from build123d import *

# Parameters (mm, degrees)
F0_R     = 2.05
F0_W     = 5.2
F0_H     = 2.15
F1_DEPTH = 2.9
F0_H_2   = 2.9
F2_DEPTH = 8


with BuildPart() as f1:
    # F0 (on Front) → F1 (new body)
    with BuildSketch(Plane.XZ):
        with BuildLine():
            Line((25.45, 4.556051), (4.65, 4.556051))
            ThreePointArc((4.65, 4.556051), (0, 6.51), (-4.65, 4.556051))
            Line((-4.65, 4.556051), (-16.95, 4.556051))
            ThreePointArc((-16.95, 4.556051), (-35.532978, 0), (-16.95, -4.556051))
            Line((-16.95, -4.556051), (-4.65, -4.556051))
            ThreePointArc((-4.65, -4.556051), (0, -6.51), (4.65, -4.556051))
            Line((4.65, -4.556051), (25.45, -4.556051))
            ThreePointArc((25.45, -4.556051), (31.693638, -7.699915), (37.907447, -4.497499))
            Line((37.907447, -4.497499), (37.907447, 0))
            Line((37.907447, 0), (37.907447, 4.497499))
            ThreePointArc((37.907447, 4.497499), (31.693638, 7.699915), (25.45, 4.556051))
        make_face()
        Polygon((-32.329781, 0), (-25.682978, 6.646804), (-19.036174, 0), (-25.682978, -6.646804), align=None, mode=Mode.SUBTRACT)
        with Locations((31.657447, 0)):
            Circle(F0_R, mode=Mode.SUBTRACT)
        Polygon((45.207447, 4.497499), (37.907447, 4.497499), (37.907447, 0), (37.907447, -4.497499), (40.007447, -4.497499), (45.207447, -4.497499), align=None)
        with Locations((42.607447, -5.572499)):
            Rectangle(F0_W, F0_H)
    extrude(amount=F1_DEPTH)

    # F0 (on Front) → F2 (join)
    with BuildSketch(Plane.XZ):
        with Locations((42.607447, -8.097499)):
            Rectangle(F0_W, F0_H_2)
    extrude(amount=F2_DEPTH)


solid = f1.part
Geometry: final body of the model. Coordinates: model frame, mm. A direction names the side the tool comes from. Coordinates: 2 decimals unless noted, no trailing zeros. Order: outer loops, then holes, each group sorted by start corner. A loop starts at its lowest first (then second) coordinate and runs counter-clockwise, first axis right, second up.
(1) Section query C-C (x = -5.5). Return the cut outline in (y, z).
(2) Section query D-D (y = -7). Return the cut outline in (x, z), plus the area to 3 significant figures.
(3) Draft query along X for faces 4 (the face through (-0.07, -1.43, -6.51)), 5 (the face through (4, -2.9, 0)), 6 (the face through (45.207, -2, -4)). Return one class per face: pulls with the +X half, pulls with the -X half, needs draft (parallel to the pull), parting line crosses it, or undercut.
(4) First-contact query: pin 1 (2.5 mm diameter, centred on x = 41, y = -1, fed in from +Z); pin 2 (8 mm diameter, centred on x = -20.5, z = 3.5, fed in from -Y); pin 3 (3 mm diameter, centred on x = -5, y = -1.5, fed in from -Z). Flat tips, straight axial feed; report the tip coordinate or a pass-through.
(5) Access query for faces 1 (the face through (42, -1, 4.497)), 2 (the face through (-29.05, -1.43, 3.28)), 3 (the face through (39, -1, -4.497)). Directions: +Z, -Z, +X, -X, +Y, -Y. A direction counts if a zero-diameter tool reaches every point of the face in a straight line with its end or side. Return the directions, or none.
(6) Section query A-A (y = -1.5). Return the cut outline in (x, z).
(7) Material intervals for probe 1 along Y at (x, z) = (-13, 1.75); probe 2 along X at (y, z) = (-2, -9); probe 3 along Z at (x, y) = (14.5, -0.75), sorted ascending.
(8) Section query B-B (z = 3). Return the cut outline in (x, y) (3 decimals).
Solution:
1. outline: (-2.9, -4.56) - (0, -4.56) - (0, 4.56) - (-2.9, 4.56) - close
2. outline: (40.01, -9.55) - (45.21, -9.55) - (45.21, -6.65) - (40.01, -6.65) - close
2. area: 15.1 mm2
3. face 4: undercut
3. face 5: needs draft
3. face 6: pulls with the +X half
4. pin 1: stops at z = 4.5
4. pin 2: stops at y = -2.9
4. pin 3: stops at z = -5.49
5. face 1: +Z, +X, +Y, -Y
5. face 2: +Y, -Y
5. face 3: -Z, +Y, -Y
6. outline: (-16.95, -4.56) - (-4.65, -4.56) arc R6.51 ccw to (4.65, -4.56) - (25.45, -4.56) arc R7.7 ccw to (37.91, -4.5) - (40.01, -4.5) - (40.01, -9.55) - (45.21, -9.55) - (45.21, 4.5) - (37.91, 4.5) arc R7.7 ccw to (25.45, 4.56) - (4.65, 4.56) arc R6.51 ccw to (-4.65, 4.56) - (-16.95, 4.56) arc R9.85 ccw (long way) to start; hole (-32.33, 0) - (-25.68, -6.65) - (-19.04, 0) - (-25.68, 6.65) - close; hole circle Ø4.1 at (31.66, 0)
7. probe 1: y = -2.9 to 0
7. probe 2: x = -29.69 to -21.68, 40.01 to 45.21
7. probe 3: z = -4.56 to 4.56
8. outline: (-35.065, -2.9) - (-29.33, -2.9) - (-29.33, 0) - (-35.065, 0) - close; (-22.036, -2.9) - (45.207, -2.9) - (45.207, 0) - (-22.036, 0) - close
